```python
from build123d import *

# Parameters (mm, degrees)
SKETCH1_W           = 121.92
SKETCH1_H           = 121.92
SKETCH1_R           = 1.27
SKETCH1_R_2         = 0.889
BOSS_EXTRUDE1_DEPTH = 5.08
FILLET1_R           = 2.54
BOSS_EXTRUDE2_START = 59.69
SKETCH3_W           = 111.76
SKETCH3_H           = 111.76
BOSS_EXTRUDE2_DEPTH = 59.69
SKETCH11_R          = 4.064
SKETCH11_R_2        = 0.889
SKETCH11_R_3        = 4.445
SKETCH11_R_4        = 1.27
BOSS_EXTRUDE5_DEPTH = 6.35
CUT_EXTRUDE1_REACH  = 152.916
SKETCH6_W           = 45.72
SKETCH6_H           = 1.143
CUT_EXTRUDE2_DEPTH  = 3.556
BOSS_EXTRUDE4_START = 6.35
SKETCH10_W          = 101.6
SKETCH10_H          = 101.6
BOSS_EXTRUDE4_DEPTH = 6.35
CHAMFER1_SIZE       = 5.08
CHAMFER2_SIZE       = 3.81
CUT_EXTRUDE3_REACH  = 151.752
SKETCH13_W          = 12.7
SKETCH13_H          = 15.24
SKETCH16_W          = 35.56
SKETCH16_H          = 22.225
SKETCH16_W_2        = 5.08
BOSS_EXTRUDE6_DEPTH = 5.08
BOSS_EXTRUDE7_REACH = 135.14
SKETCH18_R          = 6.35
SKETCH18_R_2        = 1.651
CUT_EXTRUDE4_DEPTH  = 146.823432959
SKETCH19_R          = 2.2225
CUT_EXTRUDE5_DEPTH  = 12.7


with BuildPart() as part:
    # Sketch1 → Boss-Extrude1 (new body)
    with BuildSketch(Plane.XY):
        Rectangle(SKETCH1_W, SKETCH1_H)
        with Locations((-33.909, -22.9489)):
            Circle(SKETCH1_R, mode=Mode.SUBTRACT)
        with Locations((33.909, -22.9489)):
            Circle(SKETCH1_R, mode=Mode.SUBTRACT)
        with Locations(Location((33.909, 21.6281, 0), (0, 0, 180))):
            Circle(SKETCH1_R, mode=Mode.SUBTRACT)
        with Locations(Location((-33.909, 21.6281, 0), (0, 0, 180))):
            Circle(SKETCH1_R, mode=Mode.SUBTRACT)
        with Locations((-13.208, 26.6573)):
            Circle(SKETCH1_R_2, mode=Mode.SUBTRACT)
        with Locations((52.324, 26.6573)):
            Circle(SKETCH1_R_2, mode=Mode.SUBTRACT)
        with Locations(Location((52.324, 52.4383, 0), (0, 0, 180))):
            Circle(SKETCH1_R_2, mode=Mode.SUBTRACT)
        with Locations(Location((-13.208, 52.4383, 0), (0, 0, 180))):
            Circle(SKETCH1_R_2, mode=Mode.SUBTRACT)
    extrude(amount=BOSS_EXTRUDE1_DEPTH)

    # Fillet1
    fillet1_edges = [part.edges().sort_by_distance(p)[0] for p in [
        (60.96, -60.96, 2.54),
        (-60.96, -60.96, 2.54),
        (-60.96, 60.96, 2.54),
        (60.96, 60.96, 2.54),
    ]]
    fillet(fillet1_edges, radius=FILLET1_R)

    # Sketch3 → Boss-Extrude2 (add)
    with BuildSketch(Plane.XY.offset(5.08).offset(BOSS_EXTRUDE2_START)):
        with BuildLine():
            Line((58.42, 60.96), (-58.42, 60.96))
            ThreePointArc((-58.42, 60.96), (-60.216051224, 60.216051224), (-60.96, 58.42))
            Line((-60.96, 58.42), (-60.96, -58.42))
            ThreePointArc((-60.96, -58.42), (-60.216051224, -60.216051224), (-58.42, -60.96))
            Line((-58.42, -60.96), (58.42, -60.96))
            ThreePointArc((58.42, -60.96), (60.216051224, -60.216051224), (60.96, -58.42))
            Line((60.96, -58.42), (60.96, 58.42))
            ThreePointArc((60.96, 58.42), (60.216051224, 60.216051224), (58.42, 60.96))
        make_face()
        Rectangle(SKETCH3_W, SKETCH3_H, mode=Mode.SUBTRACT)
    extrude(amount=-BOSS_EXTRUDE2_DEPTH)

    # Sketch11 → Boss-Extrude5 (add)
    # profile 1 of 8: a face of its own
    with BuildSketch(Plane.XY.offset(5.08)):
        with Locations((52.324, 52.4383)):
            Circle(SKETCH11_R)
        with Locations(Location((52.324, 52.4383, 0), (0, 0, 180))):
            Circle(SKETCH11_R_2, mode=Mode.SUBTRACT)
    # profile 2 of 8: a face of its own
    with BuildSketch(Plane.XY.offset(5.08)):
        with Locations((52.324, 26.6573)):
            Circle(SKETCH11_R)
        with Locations((52.324, 26.6573)):
            Circle(SKETCH11_R_2, mode=Mode.SUBTRACT)
    # profile 3 of 8: a face of its own
    with BuildSketch(Plane.XY.offset(5.08)):
        with Locations(Location((33.909, 21.6281, 0), (0, 0, 180))):
            Circle(SKETCH11_R_3)
        with Locations(Location((33.909, 21.6281, 0), (0, 0, 180))):
            Circle(SKETCH11_R_4, mode=Mode.SUBTRACT)
    # profile 4 of 8: a face of its own
    with BuildSketch(Plane.XY.offset(5.08)):
        with Locations((-13.208, 52.4383)):
            Circle(SKETCH11_R)
        with Locations(Location((-13.208, 52.4383, 0), (0, 0, 180))):
            Circle(SKETCH11_R_2, mode=Mode.SUBTRACT)
    # profile 5 of 8: a face of its own
    with BuildSketch(Plane.XY.offset(5.08)):
        with Locations(Location((-13.208, 26.6573, 0), (0, 0, 180))):
            Circle(SKETCH11_R)
        with Locations((-13.208, 26.6573)):
            Circle(SKETCH11_R_2, mode=Mode.SUBTRACT)
    # profile 6 of 8: a face of its own
    with BuildSketch(Plane.XY.offset(5.08)):
        with Locations(Location((-33.909, -22.9489, 0), (0, 0, 180))):
            Circle(SKETCH11_R_3)
        with Locations((-33.909, -22.9489)):
            Circle(SKETCH11_R_4, mode=Mode.SUBTRACT)
    # profile 7 of 8: a face of its own
    with BuildSketch(Plane.XY.offset(5.08)):
        with Locations(Location((-33.909, 21.6281, 0), (0, 0, 180))):
            Circle(SKETCH11_R_3)
        with Locations(Location((-33.909, 21.6281, 0), (0, 0, 180))):
            Circle(SKETCH11_R_4, mode=Mode.SUBTRACT)
    # profile 8 of 8: a face of its own
    with BuildSketch(Plane.XY.offset(5.08)):
        with Locations(Location((33.909, -22.9489, 0), (0, 0, 180))):
            Circle(SKETCH11_R_3)
        with Locations((33.909, -22.9489)):
            Circle(SKETCH11_R_4, mode=Mode.SUBTRACT)
    extrude(amount=BOSS_EXTRUDE5_DEPTH)

    # Sketch5 → Cut-Extrude1 (cut, up to next)
    with BuildSketch(Plane(origin=(60.96, 0, 0), x_dir=(0, 0, -1), z_dir=(1, 0, 0)), mode=Mode.PRIVATE) as cut_extrude1_sk1:
        with BuildLine():
            Line((-12.065, -54.61), (-57.785, -54.61))
            ThreePointArc((-57.785, -54.61), (-58.323815367, -54.386815367), (-58.547, -53.848))
            Line((-58.547, -53.848), (-58.547, -27.8638))
            ThreePointArc((-58.547, -27.8638), (-58.323815367, -27.324984633), (-57.785, -27.1018))
            Line((-57.785, -27.1018), (-12.065, -27.1018))
            ThreePointArc((-12.065, -27.1018), (-11.526184633, -27.324984633), (-11.303, -27.8638))
            Line((-11.303, -27.8638), (-11.303, -53.848))
            ThreePointArc((-11.303, -53.848), (-11.526184633, -54.386815367), (-12.065, -54.61))
        make_face()
    cut_extrude1_tool1 = extrude(cut_extrude1_sk1.sketch, amount=-CUT_EXTRUDE1_REACH, mode=Mode.PRIVATE) & part.part
    cut_extrude1 = cut_extrude1_tool1.solids().sort_by_distance((60.96, -40.8559, 34.925))[0]
    add(cut_extrude1, mode=Mode.SUBTRACT)

    # Sketch6 → Cut-Extrude2 (cut)
    with BuildSketch(Plane.ZY.offset(-55.88)):
        with Locations((34.925, -55.1815)):
            Rectangle(SKETCH6_W, SKETCH6_H)
        with Locations((34.925, -26.5303)):
            Rectangle(SKETCH6_W, SKETCH6_H)
    cut_extrude2 = extrude(amount=-CUT_EXTRUDE2_DEPTH, mode=Mode.SUBTRACT)

    # Mirror2: Cut-Extrude1, Cut-Extrude2 across plane
    add(cut_extrude1.mirror(Plane(origin=(0, 0, 0), x_dir=(0, 0, 1), z_dir=(1, 0, 0))), mode=Mode.SUBTRACT)
    add(cut_extrude2.mirror(Plane(origin=(0, 0, 0), x_dir=(0, 0, 1), z_dir=(1, 0, 0))), mode=Mode.SUBTRACT)

    # Sketch10 → Boss-Extrude4 (add)
    with BuildSketch(Plane.XY.offset(64.77).offset(BOSS_EXTRUDE4_START)):
        with BuildLine():
            Line((58.42, 60.96), (-58.42, 60.96))
            ThreePointArc((-58.42, 60.96), (-60.216051224, 60.216051224), (-60.96, 58.42))
            Line((-60.96, 58.42), (-60.96, -58.42))
            ThreePointArc((-60.96, -58.42), (-60.216051224, -60.216051224), (-58.42, -60.96))
            Line((-58.42, -60.96), (58.42, -60.96))
            ThreePointArc((58.42, -60.96), (60.216051224, -60.216051224), (60.96, -58.42))
            Line((60.96, -58.42), (60.96, 58.42))
            ThreePointArc((60.96, 58.42), (60.216051224, 60.216051224), (58.42, 60.96))
        make_face()
        Rectangle(SKETCH10_W, SKETCH10_H, mode=Mode.SUBTRACT)
    extrude(amount=-BOSS_EXTRUDE4_DEPTH)

    # Chamfer1
    chamfer1_edges = [part.edges().sort_by_distance(p)[0] for p in [
        (55.88, 0, 64.77),
        (0, 55.88, 64.77),
        (-55.88, 0, 64.77),
        (0, -55.88, 64.77),
    ]]
    chamfer(chamfer1_edges, length=CHAMFER1_SIZE - 0.0001)  # a hair under: the kernel refuses the full size

    # Chamfer2
    chamfer2_edges = [part.edges().sort_by_distance(p)[0] for p in [
        (49.530944347, 49.486192936, 5.08),
        (48.26, 26.6573, 5.08),
        (38.354, 21.6281, 5.08),
        (-13.208, 48.3743, 5.08),
        (-9.144, 26.6573, 5.08),
        (-29.464, -22.9489, 5.08),
        (-29.464, 21.6281, 5.08),
        (38.354, -22.9489, 5.08),
    ]]
    chamfer(chamfer2_edges, length=CHAMFER2_SIZE)

    # Sketch13 → Cut-Extrude3 (cut, up to next)
    with BuildSketch(Plane.ZY.offset(-55.88), mode=Mode.PRIVATE) as cut_extrude3_sk1:
        with Locations((27.559, 39.5478)):
            Rectangle(SKETCH13_W, SKETCH13_H)
    cut_extrude3_tool1 = extrude(cut_extrude3_sk1.sketch, amount=-CUT_EXTRUDE3_REACH, mode=Mode.PRIVATE) & part.part
    add(cut_extrude3_tool1.solids().sort_by_distance((55.88, 39.5478, 27.559))[0], mode=Mode.SUBTRACT)

    # Sketch16 → Boss-Extrude6 (add)
    with BuildSketch(Plane(origin=(-55.88, 0, 0), x_dir=(0, 0, -1), z_dir=(1, 0, 0))):
        with Locations((-41.91, 44.7675)):
            Rectangle(SKETCH16_W, SKETCH16_H)
        with Locations((-62.23, 44.7675)):
            Rectangle(SKETCH16_W_2, SKETCH16_H)
    extrude(amount=BOSS_EXTRUDE6_DEPTH)

    # Sketch17 → Boss-Extrude7 (add, up to next)
    with BuildSketch(Plane.XZ.offset(-33.655), mode=Mode.PRIVATE) as boss_extrude7_sk1:
        Polygon((-55.88, 24.13), (-55.88, 19.05), (-50.8, 24.13), align=None)
    boss_extrude7_tool1 = extrude(boss_extrude7_sk1.sketch, amount=-BOSS_EXTRUDE7_REACH, mode=Mode.PRIVATE) - part.part
    add(boss_extrude7_tool1.solids().sort_by_distance((-54.186667, 33.655, 22.436667))[0])

    # Sketch18 → Cut-Extrude4 (cut, through all)
    with BuildSketch(Plane(origin=(-50.8, 0, 0), x_dir=(0, 0, -1), z_dir=(1, 0, 0))):
        with Locations((-41.91, 44.7675)):
            Circle(SKETCH18_R)
        with Locations((-54.61, 44.7675)):
            Circle(SKETCH18_R_2)
        with Locations((-29.21, 44.7675)):
            Circle(SKETCH18_R_2)
    extrude(amount=-CUT_EXTRUDE4_DEPTH, mode=Mode.SUBTRACT)

    # Sketch19 → Cut-Extrude5 (cut)
    with BuildSketch(Plane.XY.offset(71.12)):
        with Locations((-55.88, -55.88)):
            Circle(SKETCH19_R)
        with Locations((-55.88, 55.88)):
            Circle(SKETCH19_R)
        with Locations((55.88, 55.88)):
            Circle(SKETCH19_R)
        with Locations((55.88, -55.88)):
            Circle(SKETCH19_R)
    extrude(amount=-CUT_EXTRUDE5_DEPTH, mode=Mode.SUBTRACT)


solid = part.part
```
The model under review builds one solid part; all positions refer to its coordinate system, in mm. A direction names the side the tool comes from. Round coordinates to 2 decimals unless told otherwise and drop trailing zeros. Use one line per item in the form item = value.
Q1. For line 1 (Y direction, x = 55.88, z = 67); line 2 (Y direction, x = 14, z = 45); line 3 (X direction, y = -26.5, z = 46), list the stretches that pass through material, from the lowest coordinate up. Write a range as [from, to].
Answer key:
line_1 = [-60.96, -58.1], [-53.66, 53.66], [58.1, 60.96]
line_2 = [-60.96, -55.88], [55.88, 60.96]
line_3 = [-60.96, -59.44], [59.44, 60.96]
Q2. Draft analysis for pull direction Z (two halves, no side actions). For faces 1 (the flat face through (1, 60.96, 36)), 2 (the conical face through (37.583, 24.445, 8.705)), 3 (the conical face through (48.08, 26.81, 8.71)), state which applies: +Z half, -Z half, draft (parallel to the pull), parting line (faces both ways), or undercut.
Answer key:
face_1 = draft
face_2 = +Z half
face_3 = undercut
Q3. Consider section A-A (y = -44). State how many separate pieces and enclosed holes the cut face has, and give its area (3 significant figures).
Answer key:
separate_pieces = 3
enclosed_holes = 0
area = 901 mm2
Q4. Insertion check: pin 1 Ø10 at (x, y) = (26.5, 18) entering from +Z; pin 2 Ø8 at (x, y) = (-25.5, 27.5) entering from +Z; pin 3 Ø1.2 at (x, z) = (-60, 36) entering from +Y. Each pin has a flat end and moves straight along its axis. Give the tip position at first contact, or say it passes through.
Answer key:
pin_1 = 11.43
pin_2 = 7.08
pin_3 = 60.76
Q5. Tool access review of faces 4 (the flat face through (50.8, -1, 68)), 5 (the conical face through (48.73, 48.83, 7.86)), 6 (the flat face through (58, 31.928, 27)): name each direction out of +Z, -Z, +X, -X, +Y, -Y from which nothing blocks a thin tool from reaching the whole face with its end or side.
Answer key:
face_4 = +Z
face_5 = none
face_6 = +X
